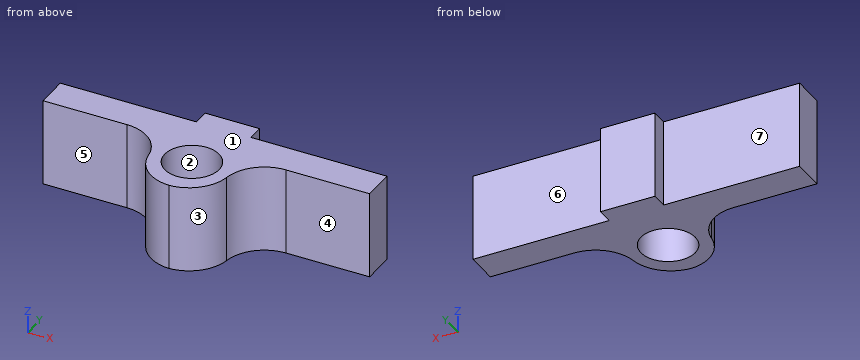
from build123d import *

# Parameters (mm, degrees)
SKETCH1_W           = 60
SKETCH1_H           = 16
BOSS_EXTRUDE1_DEPTH = 6
SKETCH2_W           = 10
SKETCH2_H           = 16
BOSS_EXTRUDE2_DEPTH = 3
SKETCH4_W           = 14.5
SKETCH4_H           = 16
BOSS_EXTRUDE3_DEPTH = 13
SKETCH5_R           = 5
CUT_EXTRUDE1_DEPTH  = 64.442887702
FILLET1_R           = 7.5
FILLET2_R           = 7.5


with BuildPart() as part:
    # Sketch1 → Boss-Extrude1 (new body)
    with BuildSketch(Plane(origin=(0, 0, 0), x_dir=(1, 0, 0), z_dir=(0, 1, 0))):
        with Locations((30, 8)):
            Rectangle(SKETCH1_W, SKETCH1_H)
    extrude(amount=BOSS_EXTRUDE1_DEPTH)

    # Sketch2 → Boss-Extrude2 (add)
    with BuildSketch(Plane(origin=(0, 6, 0), x_dir=(1, 0, 0), z_dir=(0, 1, 0))):
        with Locations((30, 8)):
            Rectangle(SKETCH2_W, SKETCH2_H)
    extrude(amount=BOSS_EXTRUDE2_DEPTH)

    # Sketch4 → Boss-Extrude3 (add)
    with BuildSketch(Plane.XZ):
        with Locations((30, -8)):
            Rectangle(SKETCH4_W, SKETCH4_H)
    extrude(amount=BOSS_EXTRUDE3_DEPTH)

    # Sketch5 → Cut-Extrude1 (cut, through all)
    with BuildSketch(Plane(origin=(0, 0, -16), x_dir=(-1, 0, 0), z_dir=(0, 0, -1))):
        with Locations((-30, -5)):
            Circle(SKETCH5_R)
    extrude(amount=-CUT_EXTRUDE1_DEPTH, mode=Mode.SUBTRACT)

    # Fillet1
    # the kernel refuses this fillet: 7.5 mm, written as the material it takes off along each edge
    with BuildSketch(Plane(origin=(22.75, -13, -34.75), x_dir=(0, 1, 0), z_dir=(0, 0, 1))) as fillet1_piece_1:
        with BuildLine():
            CenterArc((FILLET1_R, -FILLET1_R), FILLET1_R, 90, 90)
            Line((0, -FILLET1_R), (0, 0))
            Line((0, 0), (FILLET1_R, 0))
        make_face()
    extrude(amount=53.5, mode=Mode.SUBTRACT)
    with BuildSketch(Plane(origin=(37.25, -13, 18.75), x_dir=(-1, 0, 0), z_dir=(0, 0, -1))) as fillet1_piece_2:
        with BuildLine():
            CenterArc((FILLET1_R, FILLET1_R), FILLET1_R, 180, 90)
            Line((0, FILLET1_R), (0, 0))
            Line((0, 0), (FILLET1_R, 0))
        make_face()
    extrude(amount=53.5, mode=Mode.SUBTRACT)

    # Fillet2
    fillet2_edges = [part.edges().sort_by_distance(p)[0] for p in [
        (22.75, 0, -8),
        (37.25, 0, -8),
    ]]
    fillet(fillet2_edges, radius=FILLET2_R)


solid = part.part
Design review of the part built by this model. Coordinates are the model's own, in mm. Face numbers are marked on the shaded views. A direction names the side the tool comes from. Coordinates: 2 decimals unless noted, no trailing zeros. Order: outer loops, then holes, each group sorted by start corner. A loop starts at its lowest first (then second) coordinate and runs counter-clockwise, first axis right, second up. Notation, with made-up numbers: (-38.75, 0) - (-3.75, 0) arc R29 ccw to (-3.75, 34) - close; hole circle Ø5 at (-15.75, 42). An arc over 180 degrees is marked (long way). Put each result on its own line as item: value.
1) Take a section at C-C, the plane x = 53.5. Give the boundary of the cut face in (y, z), and give its area (3 significant figures).
Response values:
outline: (0, -16) - (6, -16) - (6, 0) - (0, 0) - close
area: 96.0 mm²
2) Tool access review of the marked faces 4, 5, 6 and 7: name each direction out of +Z, -Z, +X, -X, +Y, -Y from which nothing blocks a thin tool from reaching the whole face with its end or side.
Response values:
face 4: +Z, -Z, +X, -Y
face 5: +Z, -Z, -X, -Y
face 6: +Z, -Z, +X, +Y
face 7: +Z, -Z, -X, +Y
3) Wall thickness on L1, parallel to Y at x = 30, z = -6.75; L2, parallel to Y at x = 53.5, z = -14.5; L3, parallel to X at y = -2.25, z = -5.5: over which ranges is each line inside the solid? List them lowest first. Write a range as from..to.
Response values:
L1: y = -13..-10, 0..9
L2: y = 0..6
L3: x = 20.74..25.82, 34.18..39.26
4) Take a section at A-A, the plane y = -8.25. Give the boundary of the cut face in (x, z), and give its area (3 significant figures).
Response values:
outline: (23.27, -16) - (26.2, -16) - (26.2, 0) - (23.27, 0) - close; (33.8, -16) - (36.73, -16) - (36.73, 0) - (33.8, 0) - close
area: 93.7 mm²
5) Take a section at D-D, the plane y = 7. Give the boundary of the cut face in (x, z).
Response values:
outline: (25, -16) - (35, -16) - (35, 0) - (25, 0) - close
6) Insertion check: P1, Ø7.5, axis at x = 51, z = -5.5, coming from the -Y side; P2, Ø2, axis at x = 42, y = -3, coming from the -Z side; P3, Ø1.5, axis at y = 7.5, z = -7, coming from the -X side; P4, Ø1.5, axis at y = -7.5, z = -8.5, coming from the +X side. Each pin has a flat end and moves straight along its axis. Give the tip position at first contact, or say it passes through.
Response values:
P1: stops at y = 0
P2: passes through
P3: stops at x = 25
P4: stops at x = 37.15
7) Take a section at B-B, the plane x = 28. Give the boundary of the cut face in (y, z), and give its area (3 significant figures).
Response values:
outline: (-12.65, -16) - (-9.58, -16) - (-9.58, 0) - (-12.65, 0) - close; (-0.42, -16) - (9, -16) - (9, 0) - (-0.42, 0) - close
area: 200 mm²
8) The part is to be moulded in two halves that separate along X. For the marked faces 1, 2 and 3, say which applies: released by +X, released by -X, zero draft, split by the parting line, or undercut.
Response values:
face 1: zero draft
face 2: undercut
face 3: released by +X
